Geometry check sheet. Reference: the model listing, model coordinates, mm. A direction names the side the tool comes from. Coordinates: 2 decimals unless noted, no trailing zeros. Order: outer loops, then holes, each group sorted by start corner. A loop starts at its lowest first (then second) coordinate and runs counter-clockwise, first axis right, second up. Notation, with made-up numbers: (19, 41.5) -> (39, 41.5) arc R17 ccw to (39, 54.5) -> close; hole circle Ø8 at (-1, 20.25). An arc over 180 degrees is marked (long way). Answer as CSV lines item,"result". Start each with the question number.
from build123d import *

# Parameters (mm, degrees)
SKETCH1_W                      = 42.25
SKETCH1_H                      = 42.25
BOSS_EXTRUDE1_DEPTH            = 2
CUT_EXTRUDE1_REACH             = 31.942
SKETCH7_R                      = 11.25
BOSS_EXTRUDE6_DEPTH            = 37.25
BOSS_EXTRUDE6_DEPTH_BACK       = 2
SKETCH9_W                      = 4
SKETCH9_H                      = 42.25
BOSS_EXTRUDE7_DEPTH            = 4
CUT_EXTRUDE2_REACH             = 83.034
SKETCH11_W                     = 10.75
SKETCH11_H                     = 20
CUT_EXTRUDE2_DIRECTION_2_DEPTH = 82.034425555
SKETCH12_W                     = 50.25
SKETCH12_H                     = 5
BOSS_EXTRUDE8_DEPTH            = 2
FILLET2_R                      = 2
CUT_EXTRUDE4_DEPTH             = 64.084021352
CUT_EXTRUDE4_DEPTH_BACK        = 64.084021352
SKETCH13_R                     = 2
CHAMFER1_SIZE                  = 1
CUT_EXTRUDE5_REACH             = 63.924
SKETCH14_W                     = 12.88865459
SKETCH14_H                     = 5.96822717
CUT_EXTRUDE5_DIRECTION_2_DEPTH = 62.924096683
BOSS_EXTRUDE9_DEPTH            = 4


with BuildPart() as part:
    # Sketch1 → Boss-Extrude1 (new body)
    with BuildSketch(Plane(origin=(0, 0, 0), x_dir=(1, 0, 0), z_dir=(0, 1, 0))):
        Rectangle(SKETCH1_W, SKETCH1_H)
    extrude(amount=BOSS_EXTRUDE1_DEPTH)

    # Sketch7 → Cut-Extrude1 (cut, up to next)
    with BuildSketch(Plane.XZ, mode=Mode.PRIVATE) as cut_extrude1_sk1:
        with Locations(Location((0, 0, 0), (0, 0, 270))):
            Circle(SKETCH7_R)
    cut_extrude1_tool1 = extrude(cut_extrude1_sk1.sketch, amount=-CUT_EXTRUDE1_REACH, mode=Mode.PRIVATE) & part.part
    add(cut_extrude1_tool1.solids().sort_by_distance((0, 0, 0))[0], mode=Mode.SUBTRACT)

    # Sketch9 → Boss-Extrude6 (add, two sides: drawn at the far end of the back side and taken through both)
    with BuildSketch(Plane(origin=(0, 2, 0), x_dir=(1, 0, 0), z_dir=(0, 1, 0)).offset(-BOSS_EXTRUDE6_DEPTH_BACK)):
        with Locations((-23.125, 0)):
            Rectangle(SKETCH9_W, SKETCH9_H)
        with Locations((23.125, 0)):
            Rectangle(SKETCH9_W, SKETCH9_H)
    extrude(amount=BOSS_EXTRUDE6_DEPTH + BOSS_EXTRUDE6_DEPTH_BACK)

    # Sketch8 → Boss-Extrude7 (add)
    # profile 1 of 2: a face of its own
    with BuildSketch(Plane(origin=(0, 39.25, 0), x_dir=(1, 0, 0), z_dir=(0, 1, 0))):
        Polygon((-25.125, -21.125), (-25.125, 11.125), (-35.875, 11.125), (-35.875, -36.125), (-25.875, -36.125), (-25.875, -21.085491291), align=None)
        with BuildLine():
            Line((-32.867964016, -31.957386071), (-33, 7))
            ThreePointArc((-33, 7), (-30.875, 9.125), (-28.75, 7))
            Line((-28.75, 7), (-28.878451254, -32.007555956))
            ThreePointArc((-28.878451254, -32.007555956), (-30.900148895, -34.124841877), (-32.867964016, -31.957386071))
        make_face(mode=Mode.SUBTRACT)
    # profile 2 of 2: a face of its own
    with BuildSketch(Plane(origin=(0, 39.25, 0), x_dir=(1, 0, 0), z_dir=(0, 1, 0))):
        Polygon((25.875, -21.085491291), (25.125, -21.125), (25.125, 11.125), (35.875, 11.125), (35.875, -36.125), (25.875, -36.125), align=None)
        with BuildLine():
            Line((28.878451254, -32.007555956), (28.75, 7))
            ThreePointArc((28.75, 7), (30.875, 9.125), (33, 7))
            Line((33, 7), (32.867964016, -31.957386071))
            ThreePointArc((32.867964016, -31.957386071), (30.900148895, -34.124841877), (28.878451254, -32.007555956))
        make_face(mode=Mode.SUBTRACT)
    extrude(amount=-BOSS_EXTRUDE7_DEPTH)

    # Sketch11 → Cut-Extrude2 (cut, up to next)
    with BuildSketch(Plane(origin=(-25.125, 0, 0), x_dir=(0, -1, 0), z_dir=(-1, 0, 0)), mode=Mode.PRIVATE) as cut_extrude2_sk1:
        with Locations((-33.875, 0)):
            Rectangle(SKETCH11_W, SKETCH11_H)
    cut_extrude2_tool1 = extrude(cut_extrude2_sk1.sketch, amount=-CUT_EXTRUDE2_REACH, mode=Mode.PRIVATE) & part.part
    add(cut_extrude2_tool1.solids().sort_by_distance((-25.125, 33.875, 0))[0], mode=Mode.SUBTRACT)

    # Sketch11 → Cut-Extrude2 direction 2 (cut)
    with BuildSketch(Plane(origin=(-25.125, 0, 0), x_dir=(0, -1, 0), z_dir=(-1, 0, 0))):
        with Locations((-33.875, 0)):
            Rectangle(SKETCH11_W, SKETCH11_H)
    extrude(amount=CUT_EXTRUDE2_DIRECTION_2_DEPTH, mode=Mode.SUBTRACT)

    # Sketch12 → Boss-Extrude8 (add)
    with BuildSketch(Plane.XY.offset(21.125)):
        with Locations((0, 36.75)):
            Rectangle(SKETCH12_W, SKETCH12_H)
        with Locations((0, 2.5)):
            Rectangle(SKETCH12_W, SKETCH12_H)
    boss_extrude8 = extrude(amount=BOSS_EXTRUDE8_DEPTH)

    # Mirror1: Boss-Extrude8 across plane
    add(boss_extrude8.mirror(Plane.XY))

    # Fillet2
    fillet2_edges = [part.edges().sort_by_distance(p)[0] for p in [
        (-23.125, 5, -21.125),
        (23.125, 5, -21.125),
        (23.125, 34.25, -21.125),
        (-23.125, 34.25, -21.125),
        (23.125, 34.25, 21.125),
        (23.125, 5, 21.125),
        (-23.125, 5, 21.125),
        (-23.125, 34.25, 21.125),
    ]]
    fillet(fillet2_edges, radius=FILLET2_R - 0.0001)  # a hair under: the kernel refuses the full size

    # Sketch13 → Cut-Extrude4 (cut, two sides: drawn at the far end of the back side and taken through both)
    with BuildSketch(Plane.XZ.offset(-2).offset(-CUT_EXTRUDE4_DEPTH_BACK)):
        with Locations((-15.499999999, 15.5)):
            Circle(SKETCH13_R)
        with Locations((15.500000001, 15.5)):
            Circle(SKETCH13_R)
        with Locations((15.500000001, -15.5)):
            Circle(SKETCH13_R)
        with Locations((-15.499999999, -15.5)):
            Circle(SKETCH13_R)
    extrude(amount=CUT_EXTRUDE4_DEPTH + CUT_EXTRUDE4_DEPTH_BACK, mode=Mode.SUBTRACT)

    # Chamfer1
    chamfer1_edges = [part.edges().sort_by_distance(p)[0] for p in [
        (0, 39.25, 21.125),
        (0, 39.25, -21.125),
        (-21.125, 39.25, 15.5625),
        (21.125, 39.25, 0),
    ]]
    chamfer(chamfer1_edges, length=CHAMFER1_SIZE)

    # Sketch14 → Cut-Extrude5 (cut, up to next)
    with BuildSketch(Plane.XZ.offset(-35.25), mode=Mode.PRIVATE) as cut_extrude5_sk1:
        with Locations((-31.569327295, -11.445399839)):
            Rectangle(SKETCH14_W, SKETCH14_H)
    cut_extrude5_tool1 = extrude(cut_extrude5_sk1.sketch, amount=-CUT_EXTRUDE5_REACH, mode=Mode.PRIVATE) & part.part
    add(cut_extrude5_tool1.solids().sort_by_distance((-31.569327, 35.25, -11.4454))[0], mode=Mode.SUBTRACT)

    # Sketch14 → Cut-Extrude5 direction 2 (cut)
    with BuildSketch(Plane.XZ.offset(-35.25)):
        with Locations((-31.569327295, -11.445399839)):
            Rectangle(SKETCH14_W, SKETCH14_H)
    extrude(amount=CUT_EXTRUDE5_DIRECTION_2_DEPTH, mode=Mode.SUBTRACT)

    # Sketch15 → Boss-Extrude9 (add)
    with BuildSketch(Plane.XZ.offset(-35.25)):
        with BuildLine():
            Line((-25.125, 10), (-35.875, 10))
            Line((-35.875, 10), (-35.875, 14))
            Line((-35.875, 14), (-32.933785094, 14))
            ThreePointArc((-32.933785094, 14), (-30.875982387, 11.837870103), (-28.81817968, 14))
            Line((-28.81817968, 14), (-25.125, 14))
            Line((-25.125, 14), (-25.125, 10))
        make_face()
    extrude(amount=-BOSS_EXTRUDE9_DEPTH)


solid = part.part
Q1. Access from +Z, -Z, +X, -X, +Y, -Y to the whole of each face (thin tool, end or side, straight path). Record for faces 4 (the flat face through (-27, 36, 10)), 5 (the flat face through (-25.875, 37, 29)), 6 (the flat face through (9, 2, 9)), 7 (the cylindrical face through (-23.097, 5.57, 21.726)), 8 (the flat face through (23, 19, -21.125)).
Q2. Release check for a two-part mould opening along Y. For faces 1 (the flat face through (0, 34.25, -22)), 2 (the flat face through (-28, 35.25, 23)), 3 (the flat face through (0, 37, 23.125)) record: released by +Y, released by -Y, zero draft, split by the parting line, or undercut.
Q3. Sectioned sample at D-D, the plane z = 15.5. Give the number of separate pieces and of enclosed holes in the cut face, then the cut area to 3 significant figures.
Q4. Go/stop test with flat-tipped pins: pin 1 Ø3 at (x, z) = (15.5, 15.5) entering from +Y; pin 2 Ø12 at (y, z) = (13, 5.5) entering from -X (3 decimals); pin 3 Ø4.5 at (x, y) = (3.5, 36) entering from +Z (3 decimals); pin 4 Ø2 at (x, y) = (-22.5, 18.5) entering from -Z (3 decimals). Record where each tip stops, or that it passes through.
Q5. Sectioned sample at C-C, the plane x = 15.5. Record the cut outline in (y, z) (3 decimals), then the cut area to 4 significant figures.
Q6. Sectioned sample at A-A, the plane y = 19. Record the cut outline in (x, z) (3 decimals), then the cut area to 3 significant figures.
Q7. Sectioned sample at B-B, the plane x = 0. Record the cut outline in (y, z) (3 decimals), then the cut area to 3 significant figures.
Q8. Thickness scan on L1, parallel to Z at x = -15.5, y = 1.3 (3 decimals); L2, parallel to X at y = 1.55, z = -15.5 (3 decimals); L3, parallel to X at y = 7, z = -10.5 (3 decimals). Record the ranges inside material, lowest first.
Geometry results:
1,face 4,"-X, +Y"
1,face 5,"+Z, +Y, -Y"
1,face 6,"+Y"
1,face 7,"+Z, +X, -X"
1,face 8,"-Z, +X, -X"
2,face 1,"undercut"
2,face 2,"released by -Y"
2,face 3,"zero draft"
3,separate pieces,"5"
3,enclosed holes,"0"
3,area,"435 mm^2"
4,pin 1,"passes through"
4,pin 2,"stops at x = -25.125"
4,pin 3,"stops at z = 23.125"
4,pin 4,"stops at z = -21.125"
5,outline,"(0, -23.125) -> (5, -23.125) -> (5, -21.125) -> (2, -21.125) -> (2, -17.5) -> (0, -17.5) -> close; (0, -13.5) -> (2, -13.5) -> (2, 13.5) -> (0, 13.5) -> close; (0, 17.5) -> (2, 17.5) -> (2, 21.125) -> (5, 21.125) -> (5, 23.125) -> (0, 23.125) -> close; (34.25, -23.125) -> (39.25, -23.125) -> (39.25, -22.125) -> (38.25, -21.125) -> (34.25, -21.125) -> close; (34.25, 21.125) -> (38.25, 21.125) -> (39.25, 22.125) -> (39.25, 23.125) -> (34.25, 23.125) -> close"
5,area,"107.5 mm^2"
6,outline,"(-25.125, -21.125) -> (-21.125, -21.125) -> (-21.125, 21.125) -> (-25.125, 21.125) -> close; (21.125, -21.125) -> (25.125, -21.125) -> (25.125, 21.125) -> (21.125, 21.125) -> close"
6,area,"338 mm^2"
7,outline,"(0, -23.125) -> (5, -23.125) -> (5, -21.125) -> (2, -21.125) -> (2, -11.25) -> (0, -11.25) -> close; (0, 11.25) -> (2, 11.25) -> (2, 21.125) -> (5, 21.125) -> (5, 23.125) -> (0, 23.125) -> close; (34.25, -23.125) -> (39.25, -23.125) -> (39.25, -22.125) -> (38.25, -21.125) -> (34.25, -21.125) -> close; (34.25, 21.125) -> (38.25, 21.125) -> (39.25, 22.125) -> (39.25, 23.125) -> (34.25, 23.125) -> close"
7,area,"78.5 mm^2"
8,L1,"z = -23.125 to -17.5, -13.5 to 13.5, 17.5 to 23.125"
8,L2,"x = -25.125 to -17.5, -13.5 to 13.5, 17.5 to 25.125"
8,L3,"x = -25.125 to -21.125, 21.125 to 25.125"
